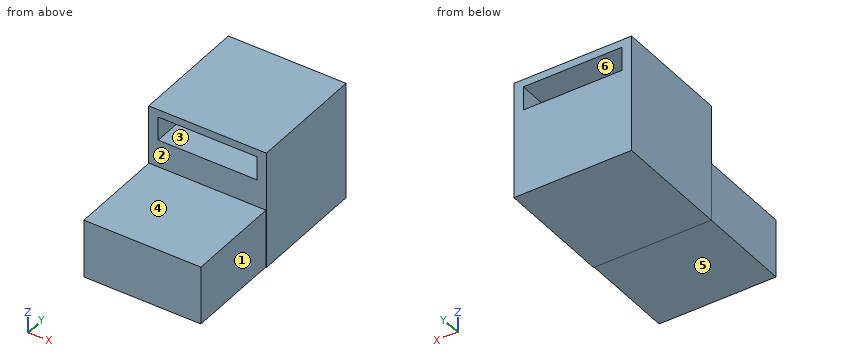
```python
from build123d import *

# Parameters (mm, degrees)
F0_W     = 127
F0_H     = 127
F0_W_2   = 106.550378
F0_H_2   = 25.665418
F1_DEPTH = 127
F2_W     = 126.253121
F2_H     = 63.126564
F3_DEPTH = 230.632


with BuildPart() as f1:
    # F0 (on Front) → F1 (new body)
    with BuildSketch(Plane.XZ):
        Rectangle(F0_W, F0_H)
        with Locations((0, 42.484045)):
            Rectangle(F0_W_2, F0_H_2, mode=Mode.SUBTRACT)
    extrude(amount=F1_DEPTH)

    # F2 (on Front) → F3 (join)
    with BuildSketch(Plane.XZ):
        with Locations((-0.129621, -31.563282)):
            Rectangle(F2_W, F2_H)
    extrude(amount=F3_DEPTH)


solid = f1.part
```
The model under review builds one solid part; all positions refer to its coordinate system, in mm. Face numbers are marked on the shaded views. A direction names the side the tool comes from. Round coordinates to 2 decimals unless told otherwise and drop trailing zeros. Loops run counter-clockwise (first coordinate to the right, second up) from the corner with the lowest first, then second, coordinate; pieces in that order, holes last. Notation, with made-up numbers: M -6,-20 L 9,-20 A16 ccw 9,4 Z; hole C 55.25,89.25 d3. An arc over 180 degrees is marked long. Put each result on its own line as item: value.
Q1. Consider section A-A, the plane x = -38. Give the boundary of the cut face in (y, z).
Result set:
outline: M -230.63,-63.13 L -127,-63.13 L -127,-63.5 L 0,-63.5 L 0,29.65 L -127,29.65 L -127,0 L -230.63,0 Z; M -127,55.32 L 0,55.32 L 0,63.5 L -127,63.5 Z
Q2. To check wall thickness, follow L1, parallel to Z at x = -14, y = -35.5; L2, parallel to X at y = -15, z = 45; L3, parallel to X at y = -181, z = -31.5. State the ranges of each line that lie inside material, in increasing order.
Result set:
L1: z = -63.5 to 29.65, 55.32 to 63.5
L2: x = -63.5 to -53.28, 53.28 to 63.5
L3: x = -63.26 to 63
Q3. Consider section D-D, the plane z = 12. Give the boundary of the cut face in (x, y).
Result set:
outline: M -63.5,-127 L 63.5,-127 L 63.5,0 L -63.5,0 Z
Q4. For pin 1 (1 mm diameter, centred on x = 25, z = 32, fed in from +Y); pin 2 (19 mm diameter, centred on y = -204.5, z = -40.5, fed in from -X); pin 3 (12 mm diameter, centred on y = -180.5, z = 3.5, fed in from +X), all flat-tipped, find the tip position at first contact; note any pin that passes through.
Result set:
pin 1: passes through
pin 2: stops at x = -63.26
pin 3: stops at x = 63
Q5. Consider section C-C, the plane y = -94. Give the boundary of the cut face in (x, z).
Result set:
outline: M -63.5,-63.5 L 63.5,-63.5 L 63.5,63.5 L -63.5,63.5 Z; hole M -53.28,29.65 L 53.28,29.65 L 53.28,55.32 L -53.28,55.32 Z
Q6. Machinability: for the marked faces 4, 5 and 6, which of the approach directions +Z, -Z, +X, -X, +Y, -Y give a long, thin tool a straight path to every point of the face, cutting with its end or side? Answer none if there is none.
Result set:
face 4: +Z, +X, -X, -Y
face 5: -Z, +X, -X, -Y
face 6: +Y, -Y
Q7. Consider section B-B, the plane z = 32. Give the boundary of the cut face in (x, y).
Result set:
outline: M -63.5,-127 L -53.28,-127 L -53.28,0 L -63.5,0 Z; M 53.28,-127 L 63.5,-127 L 63.5,0 L 53.28,0 Z
Q8. Mouldability with a two-part tool opening along X and no side actions: class the marked faces 1, 2 and 3 as released by +X, released by -X, zero draft, split by the parting line, or undercut.
Result set:
face 1: released by +X
face 2: zero draft
face 3: undercut
